Autodesk Inventor part; units mm, degrees
ref_plane "YZ Plane" through (0, 0, 0) normal (1, 0, 0) x (0, 1, 0)
ref_plane "XZ Plane" through (0, 0, 0) normal (0, 1, 0) x (-1, 0, 0)
ref_plane "XY Plane" through (0, 0, 0) normal (0, 0, 1) x (1, 0, 0)
sketch "Sketch1" plane through (0, 0, 0) normal (0, 0, 1) x (1, 0, 0)
  line L0 (-63.5, -38.1) -> (63.5, -38.1)
  line L1 (63.5, -38.1) -> (63.5, 38.1)
  line L2 (63.5, 38.1) -> (-63.5, 38.1)
  line L3 (-63.5, 38.1) -> (-63.5, -38.1)
  line L4 (-63.5, -38.1) -> (63.5, 38.1) construction
  line L5 (63.5, -38.1) -> (-63.5, 38.1) construction
  line L6 (-57.8, -32.4) -> (57.8, -32.4)
  line L7 (57.8, -32.4) -> (57.8, 32.4)
  line L8 (57.8, 32.4) -> (-57.8, 32.4)
  line L9 (-57.8, 32.4) -> (-57.8, -32.4)
  line L10 (-57.8, -32.4) -> (57.8, 32.4) construction
  line L11 (57.8, -32.4) -> (-57.8, 32.4) construction
  circle A0 centre (-57.8, 32.4) radius 1.75
  circle A1 centre (57.8, 32.4) radius 1.75
  circle A2 centre (57.8, -32.4) radius 1.75
  circle A3 centre (-57.8, -32.4) radius 1.75
  point P0 (0, 0)
  dimension "d0" = 127
  dimension "d1" = 76.2
  dimension "d2" = 115.6
  dimension "d3" = 64.8
  dimension "d4" = 3.5
extrude "Extrusion1" add sketch "Sketch1" along normal blind 2.7 contours L3 L2 L1 L0 | A3 L9 A0 L8 A1 L7 A2 L6
sketch "Sketch2" plane through (0, 0, 2.7) normal (0, 0, 1) x (1, 0, 0)
  line L0 (63.5, -38.1) -> (63.5, 38.1)
  line L1 (63.5, 38.1) -> (-63.5, 38.1)
  line L2 (-63.5, 38.1) -> (-63.5, -38.1)
  line L3 (-63.5, -38.1) -> (63.5, -38.1)
  circle A0 centre (57.8, -32.4) radius 1.75
  circle A1 centre (57.8, 32.4) radius 1.75
  circle A2 centre (-57.8, 32.4) radius 1.75
  circle A3 centre (-57.8, -32.4) radius 1.75
  line L4 (-52.1, -38.1) -> (52.1, -38.1)
  line L5 (52.1, -38.1) -> (52.1, 38.1)
  line L6 (52.1, 38.1) -> (-52.1, 38.1)
  line L7 (-52.1, 38.1) -> (-52.1, -38.1)
  line L8 (-52.1, -38.1) -> (52.1, 38.1) construction
  line L9 (52.1, -38.1) -> (-52.1, 38.1) construction
  line L10 (-63.5, -26.7) -> (63.5, -26.7)
  line L11 (63.5, -26.7) -> (63.5, 26.7)
  line L12 (63.5, 26.7) -> (-63.5, 26.7)
  line L13 (-63.5, 26.7) -> (-63.5, -26.7)
  line L14 (-63.5, -26.7) -> (63.5, 26.7) construction
  line L15 (63.5, -26.7) -> (-63.5, 26.7) construction
  point P0 (0, 0)
  point P1 (52.1, 26.7)
  point P2 (-52.1, 26.7)
  point P3 (-52.1, -26.7)
  point P4 (52.1, -26.7)
  dimension "d7" = 5.7
  dimension "d8" = 5.7
extrude "Extrusion2" add sketch "Sketch2" along normal blind 35 contours L10 L5 L12 L0 | L3 L7 L10 L5 | L10 L7 L12 L5 | L12 L7 L1 L5 | L10 L2 L12 L7
equation "\"d8\" = d7"
properties part number "EPP-400-24"
Read the model definition and answer for the solid it produces. Units are mm, in the model's axes. A direction names the side the tool comes from. Give positions to 0.01 mm unless a question says otherwise; leave off trailing zeros. Order: outer loops, then holes, each group sorted by start corner. A loop starts at its lowest first (then second) coordinate and runs counter-clockwise, first axis right, second up. Notation, with made-up numbers: (66.5, 50.5) -> (87.5, 50.5) arc R28 cw to (87.5, 89.5) -> close; hole circle Ø10 at (44.5, 20.25). An arc over 180 degrees is marked (long way). One line per item, written item: value. Start each with the question number.
(1) A tool of negligible diameter and unlimited length cuts with its end or side. For faces 4 (the flat face through (58, 26.7, 20)), 5 (the flat face through (-59, 34, 2.7)), 6 (the flat face through (-58, -26.7, 20)), from which of +Z, -Z, +X, -X, +Y, -Y can it reach the whole face along a straight path? Write none if from no direction.
(2) The part is cut by section B-B (x = 57.8). Determine the outline of the cut face in (y, z).
(3) The part is cut by section C-C (z = 20). Determine the outline of the cut face in (x, y).
(4) Flat-ended cylindrical pins translate along their axes: P1, Ø3, axis at y = 29, z = 18.5, coming from the -X side; P2, Ø5.5, axis at x = -57.5, z = 28, coming from the -Y side; P3, Ø3.5, axis at x = 57, z = 15, coming from the +Y side. Find the tip coordinate at first contact, or state that the pin passes through.
(5) The part is cut by section A-A (y = 32.4). Determine the outline of the cut face in (x, z), and give its area (3 significant figures).
(6) Straight lines are drawn through the part: L1, parallel to X at y = -32.4, z = 1; L2, parallel to X at y = 31.5, z = 27; L3, parallel to Y at x = -52.5, z = 9. For each, find the intervals that lie inside material, in ascending order.
(7) For a pull along X with two mould halves and no side action, classify faces 1 (the flat face through (-52.1, 32, 20)), 2 (the flat face through (52.1, -32, 20)), 3 (the cylindrical face through (-59.55, -32.48, 1.33)) as released by +X, released by -X, zero draft, split by the parting line, or undercut.
Taken from the geometry:
1. face 4: +Z, +X, +Y
1. face 5: +Z, -X, +Y
1. face 6: +Z, -X, -Y
2. outline: (-38.1, 0) -> (-34.15, 0) -> (-34.15, 2.7) -> (-38.1, 2.7) -> close; (-30.65, 0) -> (30.65, 0) -> (30.65, 2.7) -> (26.7, 2.7) -> (26.7, 37.7) -> (-26.7, 37.7) -> (-26.7, 2.7) -> (-30.65, 2.7) -> close; (34.15, 0) -> (38.1, 0) -> (38.1, 2.7) -> (34.15, 2.7) -> close
3. outline: (-63.5, -26.7) -> (-52.1, -26.7) -> (-52.1, -38.1) -> (52.1, -38.1) -> (52.1, -26.7) -> (63.5, -26.7) -> (63.5, 26.7) -> (52.1, 26.7) -> (52.1, 38.1) -> (-52.1, 38.1) -> (-52.1, 26.7) -> (-63.5, 26.7) -> close
4. P1: x = -52.1
4. P2: y = -26.7
4. P3: y = 26.7
5. outline: (-63.5, 0) -> (-59.55, 0) -> (-59.55, 2.7) -> (-63.5, 2.7) -> close; (-56.05, 0) -> (56.05, 0) -> (56.05, 2.7) -> (52.1, 2.7) -> (52.1, 37.7) -> (-52.1, 37.7) -> (-52.1, 2.7) -> (-56.05, 2.7) -> close; (59.55, 0) -> (63.5, 0) -> (63.5, 2.7) -> (59.55, 2.7) -> close
5. area: 3,970 mm^2
6. L1: -63.5 to -59.55, -56.05 to 56.05, 59.55 to 63.5
6. L2: -52.1 to 52.1
6. L3: -26.7 to 26.7
7. face 1: released by -X
7. face 2: released by +X
7. face 3: undercut
